Check sheet for the drawn part. Datum: minimum x, y, z corner. Units: mm. A direction names the side the tool comes from. Give positions to 0.01 mm unless a question says otherwise; leave off trailing zeros. Write each loop counter-clockwise with the first axis right and the second up, starting at its lowest first coordinate (ties: lowest second). Pieces come first, ordered by that corner, then holes. Notation, with made-up numbers: (46, 65) - (105, 65) arc R24 cw to (105, 97) - close; hole circle Ø5 at (88.5, 0). An arc over 180 degrees is marked (long way). Use a Markdown table: item, result.
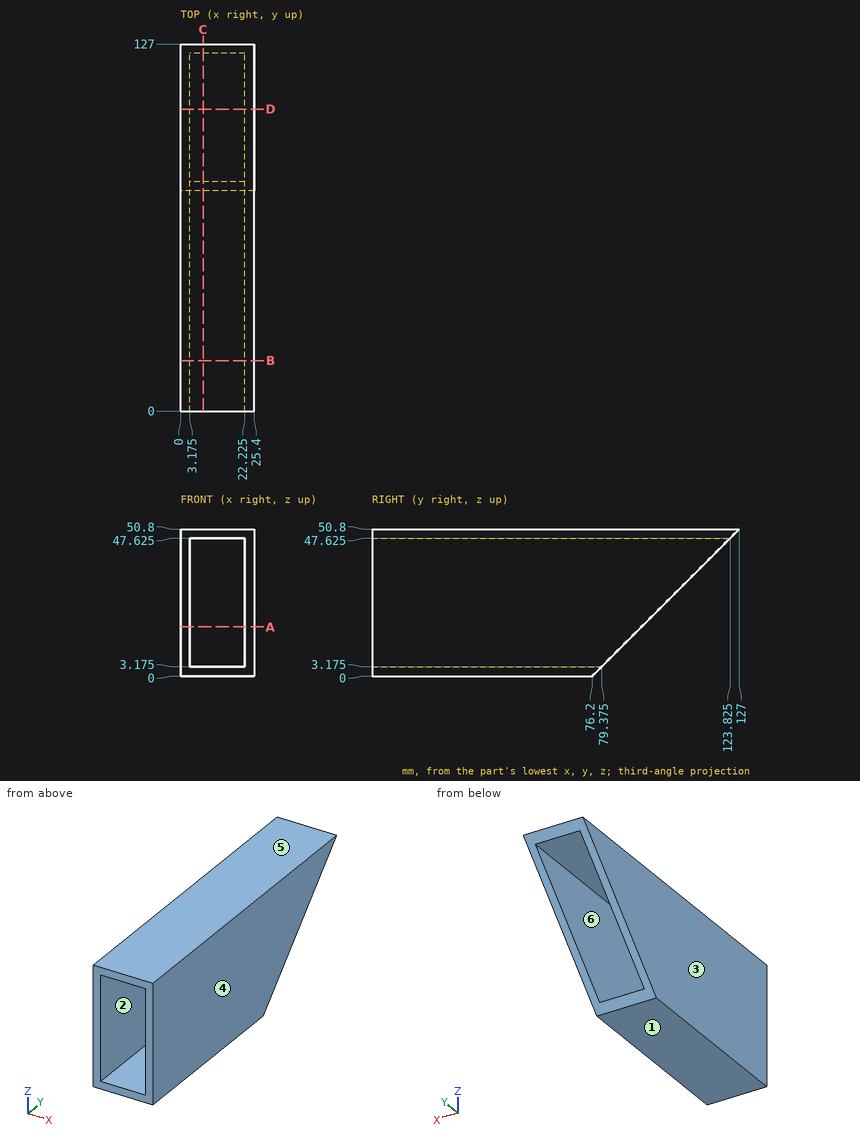
1) Section check C-C on x = 7.75. Record the boundary of the cut face in (y, z) (3 decimals).
Working result:
| item | result |
|---|---|
| outline | (0, 0) - (76.2, 0) - (79.375, 3.175) - (0, 3.175) - close; (0, 47.625) - (123.825, 47.625) - (127, 50.8) - (0, 50.8) - close |
2) Section check A-A on z = 17. Record the boundary of the cut face in (x, y) (3 decimals).
Working result:
| item | result |
|---|---|
| outline | (0, 0) - (3.175, 0) - (3.175, 93.2) - (0, 93.2) - close; (22.225, 0) - (25.4, 0) - (25.4, 93.2) - (22.225, 93.2) - close |
3) Depth check by flat-ended pin: P1, Ø3, axis at x = 13, y = 85, coming from the -Z side (3 decimals); P2, Ø5, axis at x = 11.5, y = 79.5, coming from the -Z side. Enter the tip coordinate at first touch or a pass-through.
Working result:
| item | result |
|---|---|
| P1 | stops at z = 47.625 |
| P2 | stops at z = 0.8 |
4) Section check B-B on y = 17.5. Record the boundary of the cut face in (x, z) (3 decimals), then the cut area to 3 significant figures.
Working result:
| item | result |
|---|---|
| outline | (0, 0) - (25.4, 0) - (25.4, 50.8) - (0, 50.8) - close; hole (3.175, 3.175) - (22.225, 3.175) - (22.225, 47.625) - (3.175, 47.625) - close |
| area | 444 mm² |
5) Set-up check for the marked faces 1 and 2: record each of +Z, -Z, +X, -X, +Y, -Y from which the full face is reachable in a straight line by a thin tool's end or side.
Working result:
| item | result |
|---|---|
| face 1 | -Z, +X, -X, +Y, -Y |
| face 2 | +Y, -Y |
6) Mould release check, pull along X, two halves, no side actions. Record for the marked faces 3, 4, 5 and 6: pulls with the +X half, pulls with the -X half, needs draft (parallel to the pull), parting line crosses it, or undercut.
Working result:
| item | result |
|---|---|
| face 3 | pulls with the -X half |
| face 4 | pulls with the +X half |
| face 5 | needs draft |
| face 6 | undercut |
7) Material ranges on L1, parallel to X at y = 83.5, z = 12 (3 decimals); L2, parallel to Z at x = 15.25, y = 36.5 (3 decimals); L3, parallel to Z at x = 13, y = 80 (3 decimals), recorded low to high. Write a range as from..to.
Working result:
| item | result |
|---|---|
| L1 | x = 0..3.175, 22.225..25.4 |
| L2 | z = 0..3.175, 47.625..50.8 |
| L3 | z = 47.625..50.8 |
8) Section check D-D on y = 104.5. Record the boundary of the cut face in (x, z) (3 decimals), then the cut area to 3 significant figures.
Working result:
| item | result |
|---|---|
| outline | (0, 28.3) - (3.175, 28.3) - (3.175, 47.625) - (22.225, 47.625) - (22.225, 28.3) - (25.4, 28.3) - (25.4, 50.8) - (0, 50.8) - close |
| area | 203 mm² |
